Input: part model. Units: mm. Frame: model coordinates. Face numbers are marked on the shaded views. A direction names the side the tool comes from. Give positions to 0.01 mm unless a question says otherwise; leave off trailing zeros. Loops run counter-clockwise (first coordinate to the right, second up) from the corner with the lowest first, then second, coordinate; pieces in that order, holes last. Notation, with made-up numbers: (61.25, 7.25) - (99.25, 7.25) arc R17 cw to (99.25, 29.25) - close; hole circle Ø3 at (72.25, 84). An arc over 180 degrees is marked (long way). Answer as a JSON object with one key per item and string values. Group by question number.
(1) Section query C-C (y = 18). Return loops of the section in (x, z), plus the area to 3 significant figures.
(2) Mould query, pull axis Z, two halves, no side actions, for the marked faces 1, 2 and 3. Classes: +Z half, -Z half, draft (parallel to the pull), parting line (faces both ways), or undercut.
(3) Access query for the marked faces 4, 5 and 6. Directions: +Z, -Z, +X, -X, +Y, -Y. A direction counts if a zero-diameter tool reaches every point of the face in a straight line with its end or side. Return the directions, or none.
(4) Section query D-D (x = 7). Return loops of the section in (y, z), plus the area to 3 significant figures.
(5) Material intervals for L1, parallel to Y at x = 16, z = 0; L2, parallel to Z at x = 54, y = -18.5; L3, parallel to X at y = -1.5, z = 26.5, sorted ascending.
(6) Section query A-A (z = 0). Return loops of the section in (x, y), plus the area to 3 significant figures.
(7) Section query B-B (x = 43). Return loops of the section in (y, z), plus the area to 3 significant figures.
(8) Pin query (flat end, axial travel): P1, Ø15, axis at x = 11, z = 87.5, coming from the +Y side; P2, Ø15, axis at x = 13, z = 73, coming from the -Y side; P3, Ø22.5, axis at y = 3.5, z = 70, coming from the +X side. Return the tip coordinate at first contact, or that it passes through.
```python
from build123d import *

# Parameters (mm, degrees)
SKETCH2_R           = 6
SKETCH2_R_2         = 5
BOSS_EXTRUDE3_DEPTH = 30
BOSS_EXTRUDE6_DEPTH = 12
LPATTERN1_COUNT     = 2
LPATTERN1_PITCH     = 50


with BuildPart() as part:
    # Sketch2 → Boss-Extrude3 (new body)
    with BuildSketch(Plane(origin=(0, 0, 0), x_dir=(0, 0, -1), z_dir=(1, 0, 0))):
        with BuildLine():
            Line((-101.923792087, 20.755721108), (-51.733227817, 20.755721108))
            ThreePointArc((-51.733227817, 20.755721108), (-38.793259157, 25.505894516), (-32, 37.5))
            Line((-32, 37.5), (32, 37.5))
            Line((32, 37.5), (32, -37.5))
            Line((32, -37.5), (-32, -37.5))
            ThreePointArc((-32, -37.5), (-38.41241869, -24.498337453), (-51.923792087, -19.244278892))
            Line((-51.923792087, -19.244278892), (-101.923792087, -19.244278892))
            ThreePointArc((-101.923792087, -19.244278892), (-121.923792087, 0.755721108), (-101.923792087, 20.755721108))
        make_face()
        with Locations((-101.923792087, 0.755721108)):
            Circle(SKETCH2_R, mode=Mode.SUBTRACT)
        with Locations((0, 20.755721108)):
            Circle(SKETCH2_R_2, mode=Mode.SUBTRACT)
        with Locations((0, -16.696355723)):
            Circle(SKETCH2_R_2, mode=Mode.SUBTRACT)
    extrude(amount=BOSS_EXTRUDE3_DEPTH)

    # Sketch4 → Boss-Extrude6 (add)
    with BuildSketch(Plane(origin=(0, 0, -32), x_dir=(-1, 0, 0), z_dir=(0, 0, -1))):
        with BuildLine():
            Line((-30, 37.5), (-77, 37.5))
            ThreePointArc((-77, 37.5), (-80.535533906, 36.035533906), (-82, 32.5))
            Line((-82, 32.5), (-82, -32.543310804))
            ThreePointArc((-82, -32.543310804), (-80.535533906, -36.07884471), (-77, -37.543310804))
            Line((-77, -37.543310804), (-30, -37.543310804))
            Line((-30, -37.543310804), (-30, 37.5))
        make_face()
        with BuildLine():
            Line((-59.490773049, 25.5), (-59.490773049, -25.543310804))
            ThreePointArc((-59.490773049, -25.543310804), (-64.490773049, -30.543310804), (-69.490773049, -25.543310804))
            Line((-69.490773049, -25.543310804), (-69.490773049, 25.5))
            ThreePointArc((-69.490773049, 25.5), (-64.490773049, 30.5), (-59.490773049, 25.5))
        make_face(mode=Mode.SUBTRACT)
    boss_extrude6 = extrude(amount=-BOSS_EXTRUDE6_DEPTH)

    # LPattern1: Boss-Extrude6 ×2
    with Locations(*[(0, 0, i * LPATTERN1_PITCH) for i in range(1, LPATTERN1_COUNT)]):
        add(boss_extrude6)


solid = part.part
```
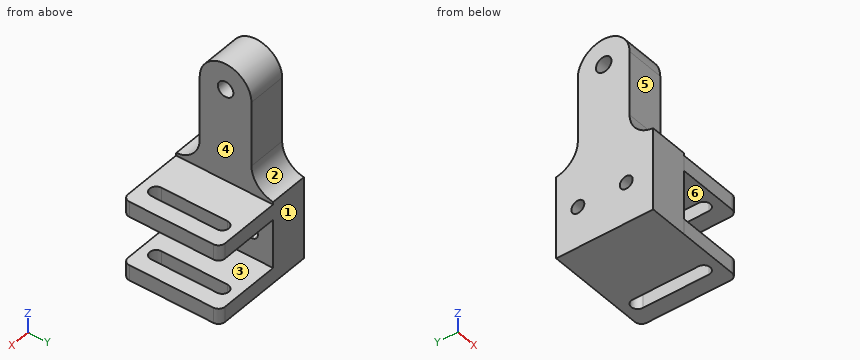
Recorded:
{
 "1": {"outline": "(0, -32) - (59.49, -32) - (59.49, -20) - (30, -20) - (30, -4.17) - (0, -4.17) - close; (0, 4.17) - (30, 4.17) - (30, 18) - (59.49, 18) - (59.49, 30) - (30, 30) - (30, 112.05) - (0, 112.05) - close; (69.49, -32) - (82, -32) - (82, -20) - (69.49, -20) - close; (69.49, 18) - (82, 18) - (82, 30) - (69.49, 30) - close", "area": "5,080 mm^2"},
 "2": {"face 1": "draft", "face 2": "+Z half", "face 3": "undercut"},
 "3": {"face 4": "+Z, +X, +Y, -Y", "face 5": "+Z, +X, -X, -Y", "face 6": "+X, +Y, -Y"},
 "4": {"outline": "(-37.5, -32) - (37.5, -32) - (37.5, 32) arc R20 cw to (20.76, 51.73) - (20.76, 101.92) arc R20 ccw to (-19.24, 101.92) - (-19.24, 51.92) arc R20 cw to (-37.5, 32) - close; hole circle Ø10 at (-16.7, 0); hole circle Ø12 at (0.76, 101.92); hole circle Ø10 at (20.76, 0)", "area": "8,120 mm^2"},
 "5": {"L1": "y = -37.5 to -21.7, -11.7 to 15.76, 25.76 to 37.5", "L2": "z = -32 to -20, 18 to 30", "L3": "x = 0 to 59.49, 69.49 to 82"},
 "6": {"outline": "(0, -37.5) - (30, -37.5) - (30, -21.7) - (0, -21.7) - close; (0, -11.7) - (30, -11.7) - (30, 15.76) - (0, 15.76) - close; (0, 25.76) - (30, 25.76) - (30, 37.5) - (0, 37.5) - close", "area": "1,650 mm^2"},
 "7": {"outline": "(-37.54, -32) - (37.5, -32) - (37.5, -20) - (-37.54, -20) - close; (-37.54, 18) - (37.5, 18) - (37.5, 30) - (-37.54, 30) - close", "area": "1,800 mm^2"},
 "8": {"P1": "stops at y = 20.76", "P2": "stops at y = -19.24", "P3": "stops at x = 30"}
}
